For this review, take the finished solid that the model builds, in its own axes (mm). Face numbers are marked on the shaded views. A direction names the side the tool comes from. Coordinates: 2 decimals unless noted, no trailing zeros. Loops run counter-clockwise (first coordinate to the right, second up) from the corner with the lowest first, then second, coordinate; pieces in that order, holes last.
1. Take a section at C-C, the plane z = -4.25. State the section outline as (x, y) points.
2. To check wall thickness, follow probe 1 along X at (y, z) = (3.5, -4.25); probe 2 along Y at (x, z) = (-8.5, -5); probe 3 along Y at (x, z) = (-4.75, -4). State the ranges of each line that lie inside material, in increasing order.
3. Mouldability with a two-part tool opening along Z and no side actions: class the marked faces 1, 2 and 3 as pulls with the +Z half, pulls with the -Z half, needs draft (parallel to the pull), parting line crosses it, or undercut.
4. Machinability: for the marked faces 4 and 5, which of the approach directions +Z, -Z, +X, -X, +Y, -Y give a long, thin tool a straight path to every point of the face, cutting with its end or side? Answer none if there is none.
5. Clearance check with flat-ended pins moving along their axes: P1, Ø3.5, axis at x = 0, y = 1.5, coming from the -Z side; P2, Ø3.5, axis at y = -3.5, z = -5, coming from the +X side; P3, Ø2.5, axis at y = 0, z = -4, coming from the -X side; P4, Ø1.5, axis at x = -5.5, z = -4, coming from the -Y side. State where each tip first meets the part, or that it passes through.
6. Take a section at B-B, the plane z = -3.25. State the section outline as (x, y) points, then the cut area to 3 significant figures.
7. Take a section at A-A, the plane z = -0.25. State the section outline as (x, y) points, then the cut area to 3 significant figures.
```python
from build123d import *

# Parameters (mm, degrees)
ESQUISSE2_W             = 20
ESQUISSE2_H             = 15
BOSS_EXTRU_1_DEPTH      = 1.5
ESQUISSE3_R             = 1.7
BOSS_EXTRU_2_DEPTH      = 20
ENL_V_MAT_EXTRU_2_DEPTH = 3.5
ENL_V_MAT_EXTRU_4_DEPTH = 21


with BuildPart() as part:
    # Esquisse2 → Boss.-Extru.1 (new body)
    with BuildSketch(Plane.XY):
        Rectangle(ESQUISSE2_W, ESQUISSE2_H)
    extrude(amount=BOSS_EXTRU_1_DEPTH)

    # Esquisse3 → Boss.-Extru.2 (add)
    with BuildSketch(Plane.ZY.offset(10)):
        with BuildLine():
            Line((-5.931892952, 2.136705913), (0, 7.5))
            Line((0, 7.5), (0, -7.5))
            Line((0, -7.5), (-5.931892952, -2.136705913))
            ThreePointArc((-5.931892952, -2.136705913), (-6.880576771, 0), (-5.931892952, 2.136705913))
        make_face()
        with Locations((-4, 0)):
            Circle(ESQUISSE3_R, mode=Mode.SUBTRACT)
    extrude(amount=-BOSS_EXTRU_2_DEPTH)

    # Esquisse5 → Enlèv. mat.-Extru.2 (cut, symmetric)
    with BuildSketch(Plane.ZY):
        with BuildLine():
            Line((0.421634759, 7.5), (0.421634759, -7.5))
            Line((0.421634759, -7.5), (0, -7.5))
            Line((0, -7.5), (-5.931892952, -2.136705913))
            ThreePointArc((-5.931892952, -2.136705913), (-6.880576771, 0), (-5.931892952, 2.136705913))
            Line((-5.931892952, 2.136705913), (0, 7.5))
            Line((0, 7.5), (0.421634759, 7.5))
        make_face()
    extrude(amount=ENL_V_MAT_EXTRU_2_DEPTH, both=True, mode=Mode.SUBTRACT)

    # Esquisse4 → Enlèv. mat.-Extru.4 (cut)
    with BuildSketch(Plane.ZY.offset(10)):
        Polygon((1.222110979, 7.02363184), (1.5, 6.681425034), (1.5, 7.301520861), align=None)
        Polygon((1.222110979, 6.455765268), (1.5, 6.113558462), (1.5, 6.681425034), align=None)
        Polygon((1.222110979, 5.835669441), (1.5, 5.55778042), (1.5, 6.113558462), align=None)
        Polygon((1.222110979, 5.279891399), (1.5, 5.002002378), (1.5, 5.55778042), align=None)
        Polygon((1.222110979, 4.724113357), (1.5, 4.446224336), (1.5, 5.002002378), align=None)
        Polygon((1.222110979, 4.168335315), (1.5, 3.890446294), (1.5, 4.446224336), align=None)
        Polygon((1.222110979, 3.612557273), (1.5, 3.334668252), (1.5, 3.890446294), align=None)
        Polygon((1.222110979, 3.056779231), (1.5, 2.77889021), (1.5, 3.334668252), align=None)
        Polygon((1.222110979, 2.501001189), (1.5, 2.223112168), (1.5, 2.77889021), align=None)
        Polygon((1.222110979, 1.945223147), (1.5, 1.667334126), (1.5, 2.223112168), align=None)
        Polygon((1.222110979, 1.389445105), (1.5, 1.111556084), (1.5, 1.667334126), align=None)
        Polygon((1.222110979, 0.833667063), (1.5, 0.555778042), (1.5, 1.111556084), align=None)
        Polygon((1.222110979, 0.277889021), (1.5, 0), (1.5, 0.555778042), align=None)
        Polygon((1.5, -0.555778042), (1.5, 0), (1.222110979, -0.277889021), align=None)
        Polygon((1.5, -1.111556084), (1.5, -0.555778042), (1.222110979, -0.833667063), align=None)
        Polygon((1.5, -1.667334126), (1.5, -1.111556084), (1.222110979, -1.389445105), align=None)
        Polygon((1.5, -2.223112168), (1.5, -1.667334126), (1.222110979, -1.945223147), align=None)
        Polygon((1.5, -2.77889021), (1.5, -2.223112168), (1.222110979, -2.501001189), align=None)
        Polygon((1.5, -3.334668252), (1.5, -2.77889021), (1.222110979, -3.056779231), align=None)
        Polygon((1.5, -3.890446294), (1.5, -3.334668252), (1.222110979, -3.612557273), align=None)
        Polygon((1.5, -4.446224336), (1.5, -3.890446294), (1.222110979, -4.168335315), align=None)
        Polygon((1.5, -5.002002378), (1.5, -4.446224336), (1.222110979, -4.724113357), align=None)
        Polygon((1.5, -5.55778042), (1.5, -5.002002378), (1.222110979, -5.279891399), align=None)
        Polygon((1.5, -6.113558462), (1.5, -5.55778042), (1.222110979, -5.835669441), align=None)
        Polygon((1.5, -6.681425034), (1.5, -6.113558462), (1.222110979, -6.455765268), align=None)
        Polygon((1.5, -7.301520861), (1.5, -6.681425034), (1.222110979, -7.02363184), align=None)
    extrude(amount=-ENL_V_MAT_EXTRU_4_DEPTH, mode=Mode.SUBTRACT)


solid = part.part
```
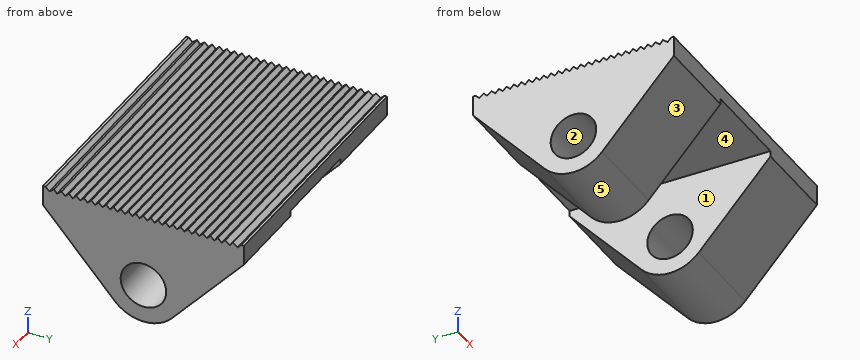
Results list:
1. outline: (-10, -3.66) - (-3.5, -3.66) - (-3.5, -1.68) - (-10, -1.68) - close; (-10, 1.68) - (-3.5, 1.68) - (-3.5, 3.66) - (-10, 3.66) - close; (3.5, -3.66) - (10, -3.66) - (10, -1.68) - (3.5, -1.68) - close; (3.5, 1.68) - (10, 1.68) - (10, 3.66) - (3.5, 3.66) - close
2. probe 1: x = -10 to -3.5, 3.5 to 10
2. probe 2: y = -2.98 to -1.37, 1.37 to 2.98
2. probe 3: y = -3.88 to -1.7, 1.7 to 3.88
3. face 1: needs draft
3. face 2: undercut
3. face 3: pulls with the -Z half
4. face 4: -Z, +Y, -Y
4. face 5: -Z, +X, -X
5. P1: stops at z = 0.42
5. P2: stops at x = 10
5. P3: passes through
5. P4: stops at y = -4.56
6. outline: (-10, -4.56) - (-3.5, -4.56) - (-3.5, -1.53) - (-10, -1.53) - close; (-10, 1.53) - (-3.5, 1.53) - (-3.5, 4.56) - (-10, 4.56) - close; (3.5, -4.56) - (10, -4.56) - (10, -1.53) - (3.5, -1.53) - close; (3.5, 1.53) - (10, 1.53) - (10, 4.56) - (3.5, 4.56) - close
6. area: 78.9 mm2
7. outline: (-10, -7.27) - (-3.5, -7.27) - (-3.5, 7.27) - (-10, 7.27) - close; (3.5, -7.27) - (10, -7.27) - (10, 7.27) - (3.5, 7.27) - close
7. area: 189 mm2
